from build123d import *

# Parameters (mm, degrees)
SKETCH8_W                   = 6.35
SKETCH8_H                   = 38.1
SKETCH8_W_2                 = 22.225
BOSS_EXTRUDE2_DEPTH         = 6.35
BOSS_EXTRUDE3_START         = 6.35
SKETCH8_3_W                 = 6.35
SKETCH8_3_H                 = 38.1
BOSS_EXTRUDE3_DEPTH         = 26.9875
F_1_4_0_25_DIAMETER_HOLE2_D = 6.35
F_1_4_20_TAPPED_HOLE1_D     = 5.1054
F_1_4_20_TAPPED_HOLE1_DEPTH = 16.51
F_1_4_20_TAPPED_HOLE1_TIP   = 1.533816902
FILLET1_R                   = 6.35
FILLET2_R                   = 6.35


with BuildPart() as part:
    # Sketch8 → Boss-Extrude2 (new body)
    with BuildSketch(Plane(origin=(0, 0, 0), x_dir=(1, 0, 0), z_dir=(0, 1, 0))):
        with Locations((-11.1125, 0)):
            Rectangle(SKETCH8_W, SKETCH8_H)
        with Locations((3.175, 0)):
            Rectangle(SKETCH8_W_2, SKETCH8_H)
    extrude(amount=BOSS_EXTRUDE2_DEPTH)

    # Sketch8<3> → Boss-Extrude3 (add)
    with BuildSketch(Plane(origin=(0, 0, 0), x_dir=(1, 0, 0), z_dir=(0, 1, 0)).offset(BOSS_EXTRUDE3_START)):
        with Locations((-11.1125, 0)):
            Rectangle(SKETCH8_3_W, SKETCH8_3_H)
    extrude(amount=BOSS_EXTRUDE3_DEPTH)

    # 1/4 (0.25) Diameter Hole2 (through all)
    with Locations(Plane(origin=(0, 6.35, 0), x_dir=(1, 0, 0), z_dir=(0, 1, 0))):
        with Locations((3.175, -9.525), (3.175, 9.525)):
            Hole(F_1_4_0_25_DIAMETER_HOLE2_D / 2)

    # 1/4-20 Tapped Hole1
    with Locations(Plane(origin=(-7.9375, 0, 0), x_dir=(0, 0, -1), z_dir=(1, 0, 0))):
        with Locations((0, 26.9875)):
            Hole(F_1_4_20_TAPPED_HOLE1_D / 2, depth=F_1_4_20_TAPPED_HOLE1_DEPTH)
            with Locations((0, 0, -(F_1_4_20_TAPPED_HOLE1_DEPTH + F_1_4_20_TAPPED_HOLE1_TIP / 2))):  # 118° drill point
                Cone(0, F_1_4_20_TAPPED_HOLE1_D / 2, F_1_4_20_TAPPED_HOLE1_TIP, mode=Mode.SUBTRACT)

    # Fillet1
    fillet1_edges = [part.edges().sort_by_distance(p)[0] for p in [
        (14.2875, 3.175, -19.05),
        (14.2875, 3.175, 19.05),
    ]]
    fillet(fillet1_edges, radius=FILLET1_R)

    # Fillet2
    fillet2_edges = [part.edges().sort_by_distance(p)[0] for p in [
        (-11.1125, 33.3375, 19.05),
        (-11.1125, 33.3375, -19.05),
    ]]
    fillet(fillet2_edges, radius=FILLET2_R)


solid = part.part
Geometry check sheet. Reference: the model listing, model coordinates, mm. A direction names the side the tool comes from. Give positions to 0.01 mm unless a question says otherwise; leave off trailing zeros. Loops run counter-clockwise (first coordinate to the right, second up) from the corner with the lowest first, then second, coordinate; pieces in that order, holes last. Notation, with made-up numbers: M 76,89.25 L 116,89.25 A27 ccw 116,122.25 Z; hole C 58.5,77.5 d4. An arc over 180 degrees is marked long. Write each question's results on one line, items separated by ' | '.
1) Section check A-A, the plane z = 0. Record the boundary of the cut face in (x, y), plus the area to 3 significant figures.
Answers follow:
outline: M -14.29,0 L 14.29,0 L 14.29,6.35 L -7.94,6.35 L -7.94,24.43 L -14.29,24.43 Z; M -14.29,29.54 L -7.94,29.54 L -7.94,33.34 L -14.29,33.34 Z | area: 320 mm2
2) Gauge pin test, flat ends, axial feed: pin 1 (5.5 mm diameter, centred on x = 3.175, z = 9.525, fed in from -Y); pin 2 (13.5 mm diameter, centred on y = 22.5, z = -5, fed in from +X). Record the tip position at first contact, or that the pin passes through.
Answers follow:
pin 1: through | pin 2: x = -7.94
3) Section check C-C, the plane y = 25. Record the boundary of the cut face in (x, z).
Answers follow:
outline: M -14.29,-19.05 L -7.94,-19.05 L -7.94,-1.6 L -14.29,-1.6 Z; M -14.29,1.6 L -7.94,1.6 L -7.94,19.05 L -14.29,19.05 Z
4) Thickness scan on line 1 (X direction, y = 12, z = 16); line 2 (Y direction, x = 5, z = -14.5); line 3 (X direction, y = 4, z = -8.5). Record the ranges inside material, lowest first.
Answers follow:
line 1: -14.29 to -7.94 | line 2: 0 to 6.35 | line 3: -14.29 to 0.17, 6.18 to 14.29
5) Section check D-D, the plane x = 4.75. Record the boundary of the cut face in (y, z).
Answers follow:
outline: M 0,-19.05 L 6.35,-19.05 L 6.35,-12.28 L 0,-12.28 Z; M 0,-6.77 L 6.35,-6.77 L 6.35,6.77 L 0,6.77 Z; M 0,12.28 L 6.35,12.28 L 6.35,19.05 L 0,19.05 Z
6) Tool access check on faces 4 (the face through (-11.157, 24.496, -0.553)), 5 (the face through (3, 6.35, 0)). Record the directions out of +Z, -Z, +X, -X, +Y, -Y that give a thin tool (end or side, any length) a straight path to the whole face; none if there is none.
Answers follow:
face 4: +X, -X | face 5: +Z, -Z, +X, +Y
7) Release check for a two-part mould opening along X. For faces 1 (the face through (1.468, 3.131, -12.202)), 2 (the face through (14.288, 3, 0)), 3 (the face through (-11.068, 31.527, -17.14)) record: +X half, -X half, draft (parallel to the pull), parting line (faces both ways), or undercut.
Answers follow:
face 1: undercut | face 2: +X half | face 3: draft
8) Section check B-B, the plane x = -12.5. Record the boundary of the cut face in (y, z).
Answers follow:
outline: M 0,-19.05 L 26.99,-19.05 A6.35 ccw 33.34,-12.7 L 33.34,12.7 A6.35 ccw 26.99,19.05 L 0,19.05 Z; hole C 26.99,0 d5.11
